```python
from build123d import *

# Parameters (mm, degrees)
F1_DEPTH = 76.2


with BuildPart() as f1:
    # F0 (on Front) → F1 (new body)
    with BuildSketch(Plane.XZ):
        with BuildLine():
            Line((-6.35, 0), (0, 0))
            Line((0, 0), (6.35, 0))
            Line((6.35, 0), (6.35, 19.05))
            Line((6.35, 19.05), (21.153298, 19.05))
            Line((21.153298, 19.05), (21.153298, 15.494))
            ThreePointArc((21.153298, 15.494), (25.459427, 21.784573), (31.75, 26.090702))
            ThreePointArc((31.75, 26.090702), (29.40245, 39.080351), (31.75, 52.07))
            ThreePointArc((31.75, 52.07), (27.94, 55.88), (24.13, 52.07))
            ThreePointArc((24.13, 52.07), (25.806343, 46.527676), (24.13, 40.985351))
            ThreePointArc((24.13, 40.985351), (24.520495, 28.555752), (14.77733, 20.828))
            Line((14.77733, 20.828), (4.572, 20.828))
            Line((4.572, 20.828), (4.572, 1.778))
            Line((4.572, 1.778), (0, 1.778))
            Line((0, 1.778), (-4.572, 1.778))
            Line((-4.572, 1.778), (-4.572, 20.828))
            Line((-4.572, 20.828), (-14.77733, 20.828))
            ThreePointArc((-14.77733, 20.828), (-24.520495, 28.555752), (-24.13, 40.985351))
            ThreePointArc((-24.13, 40.985351), (-25.806343, 46.527676), (-24.13, 52.07))
            ThreePointArc((-24.13, 52.07), (-27.94, 55.88), (-31.75, 52.07))
            ThreePointArc((-31.75, 52.07), (-29.40245, 39.080351), (-31.75, 26.090702))
            ThreePointArc((-31.75, 26.090702), (-25.459427, 21.784573), (-21.153298, 15.494))
            Line((-21.153298, 15.494), (-21.153298, 19.05))
            Line((-21.153298, 19.05), (-6.35, 19.05))
            Line((-6.35, 19.05), (-6.35, 0))
        make_face()
    extrude(amount=F1_DEPTH)


solid = f1.part
```
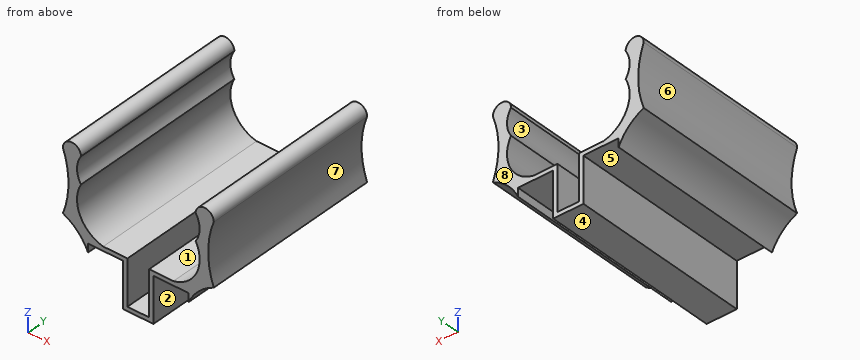
Design review of the part built by this model. Coordinates are the model's own, in mm. Face numbers are marked on the shaded views. A direction names the side the tool comes from. Give positions to 0.01 mm unless a question says otherwise; leave off trailing zeros. Order: outer loops, then holes, each group sorted by start corner. A loop starts at its lowest first (then second) coordinate and runs counter-clockwise, first axis right, second up. Notation, with made-up numbers: (33.5, 54) - (89.5, 54) arc R20 ccw to (89.5, 86) - close; hole circle Ø11 at (69, 73). An arc over 180 degrees is marked (long way). Use a Markdown table: item, result. Add a question column.
(1) Add section A-A on z = 12.5. Give the boundary of the cut face in (x, y).
(2) Add section C-C on x = 3.5. Give the boundary of the cut face in (y, z).
(3) Mouldability with a two-part tool opening along X and no side actions: class the marked faces 5, 6, 7 and 8 as +X half, -X half, draft (parallel to the pull), parting line (faces both ways), or undercut.
(4) Machinability: for the marked faces 1, 2, 3 and 4, which of the approach directions +Z, -Z, +X, -X, +Y, -Y give a long, thin tool a straight path to every point of the face, cutting with its end or side? Answer none if there is none.
(5) Add section D-D on z = 28. Give the boundary of the cut face in (x, y), then the cut area to 3 significant figures.
(6) Add section B-B on y = -65.5. Give the boundary of the cut face in (x, z).
(7) Wall thickness on probe 1 along X at (y, z) = (-38, 13.5); probe 2 along X at (y, z) = (-67.5, 28.5); probe 3 along Z at (x, y) = (-9, -23.5): over which ranges is each line inside the solid? List them lowest first. Write a range as [from, to].
(8) Clearance check with flat-ended pins moving along their axes: P1, Ø6, axis at x = 7.5, y = -65, coming from the +Z side; P2, Ø10, axis at y = -23, z = 35.5, coming from the +X side; P3, Ø4.5, axis at x = 11, y = -36.5, coming from the -Z side; P4, Ø1.5, axis at x = 2, y = -51, coming from the -Z side. State where each tip first meets the part, or that it passes through.
Report:
| question | item | result |
|---|---|---|
| 1 | outline | (-6.35, -76.2) - (-4.57, -76.2) - (-4.57, 0) - (-6.35, 0) - close; (4.57, -76.2) - (6.35, -76.2) - (6.35, 0) - (4.57, 0) - close |
| 2 | outline | (-76.2, 0) - (0, 0) - (0, 1.78) - (-76.2, 1.78) - close |
| 3 | face 5 | undercut |
| 3 | face 6 | -X half |
| 3 | face 7 | +X half |
| 3 | face 8 | draft |
| 4 | face 1 | +Z, +Y, -Y |
| 4 | face 2 | -Z, +Y, -Y |
| 4 | face 3 | +Y, -Y |
| 4 | face 4 | -Z, +X, -X, +Y, -Y |
| 5 | outline | (-31.1, -76.2) - (-24.25, -76.2) - (-24.25, 0) - (-31.1, 0) - close; (24.25, -76.2) - (31.1, -76.2) - (31.1, 0) - (24.25, 0) - close |
| 5 | area | 1,040 mm² |
| 6 | outline | (-31.75, 26.09) arc R20.71 cw to (-21.15, 15.49) - (-21.15, 19.05) - (-6.35, 19.05) - (-6.35, 0) - (6.35, 0) - (6.35, 19.05) - (21.15, 19.05) - (21.15, 15.49) arc R20.71 cw to (31.75, 26.09) arc R37.11 cw to (31.75, 52.07) arc R3.81 ccw to (24.13, 52.07) arc R10 cw to (24.13, 40.99) arc R13.84 cw to (14.78, 20.83) - (4.57, 20.83) - (4.57, 1.78) - (-4.57, 1.78) - (-4.57, 20.83) - (-14.78, 20.83) arc R13.84 cw to (-24.13, 40.99) arc R10 cw to (-24.13, 52.07) arc R3.81 ccw to (-31.75, 52.07) arc R37.11 cw to start |
| 7 | probe 1 | x = [-6.35, -4.57], [4.57, 6.35] |
| 7 | probe 2 | x = [-30.94, -24.49], [24.49, 30.94] |
| 7 | probe 3 | z = [19.05, 20.83] |
| 8 | P1 | stops at z = 20.83 |
| 8 | P2 | stops at x = 30.41 |
| 8 | P3 | stops at z = 19.05 |
| 8 | P4 | stops at z = 0 |
